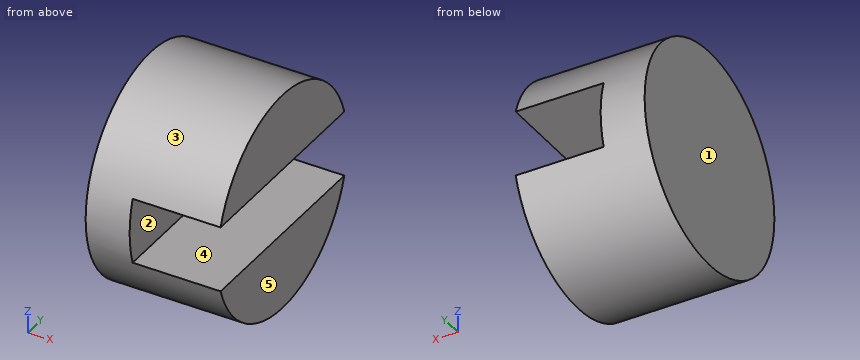
```python
from build123d import *

# Parameters (mm, degrees)
SKETCH2_R           = 5
BOSS_EXTRUDE1_DEPTH = 6
CUT_EXTRUDE1_START  = -4
CUT_EXTRUDE1_DEPTH  = 4


with BuildPart() as part:
    # Sketch2 → Boss-Extrude1 (new body)
    with BuildSketch(Plane(origin=(0, 0, 0), x_dir=(0, 0, -1), z_dir=(1, 0, 0))):
        Circle(SKETCH2_R)
    extrude(amount=BOSS_EXTRUDE1_DEPTH)

    # Sketch3 → Cut-Extrude1 (cut)
    with BuildSketch(Plane(origin=(6, 0, 0), x_dir=(0, 0, -1), z_dir=(1, 0, 0)).offset(CUT_EXTRUDE1_START)):
        with BuildLine():
            Line((-1.5, 4.769696007), (-1.5, -4.769696007))
            ThreePointArc((-1.5, -4.769696007), (0, -5), (1.5, -4.769696007))
            Line((1.5, -4.769696007), (1.5, 4.769696007))
            ThreePointArc((1.5, 4.769696007), (0, 5), (-1.5, 4.769696007))
        make_face()
    extrude(amount=CUT_EXTRUDE1_DEPTH, mode=Mode.SUBTRACT)


solid = part.part
```
Verification items for the finished model (mm, model axes). Face numbers are marked on the shaded views. A direction names the side the tool comes from. Coordinates: 2 decimals unless noted, no trailing zeros. Write each loop counter-clockwise with the first axis right and the second up, starting at its lowest first coordinate (ties: lowest second). Pieces come first, ordered by that corner, then holes. Notation, with made-up numbers: (-12, -25) - (-3, -25) arc R27 cw to (-3, 6) - close; hole circle Ø1 at (20.5, -38). An arc over 180 degrees is marked (long way). One line per question, with ' | ' between items. Start each with the question number.
1. Section check C-C (z = 0). Enter the section's corners in (x, y).
2. Section check D-D (y = 3). Enter the section's corners in (x, z), plus the area to 3 significant figures.
3. Material ranges on line 1 along Z through (x, y) = (5.1, 0); line 2 along X through (y, z) = (3.5, -1); line 3 along Y through (x, z) = (1.25, -1.5), recorded low to high.
4. Gauge pin test, flat ends, axial feed: P1, Ø1.5, axis at x = 4.5, y = -3.5, coming from the -Z side; P2, Ø3, axis at x = 4.5, y = -2, coming from the +Z side; P3, Ø1, axis at x = 3, z = 3.5, coming from the +Y side. Record the tip position at first contact, or that the pin passes through.
5. Draft check along Z on the marked faces 1, 2 and 3. Enter one of: released by +Z, released by -Z, zero draft, split by the parting line, or undercut.
6. Section check B-B (x = 3.35). Enter the section's corners in (y, z), plus the area to 3 significant figures.
7. Access from +Z, -Z, +X, -X, +Y, -Y to the whole of each face (thin tool, end or side, straight path). Record for the marked faces 4 and 5.
8. Section check A-A (y = -4). Enter the section's corners in (x, z), plus the area to 3 significant figures.
Computed values:
1) outline: (0, -5) - (2, -5) - (2, 5) - (0, 5) - close
2) outline: (0, -4) - (6, -4) - (6, -1.5) - (2, -1.5) - (2, 1.5) - (6, 1.5) - (6, 4) - (0, 4) - close | area: 36.0 mm²
3) line 1: -5 to -1.5, 1.5 to 5 | line 2: 0 to 2 | line 3: -4.77 to 4.77
4) P1: z = -4.18 | P2: z = 4.97 | P3: y = 4
5) face 1: zero draft | face 2: undercut | face 3: split by the parting line
6) outline: (-4.77, -1.5) arc R5 ccw to (4.77, -1.5) - close; (-4.77, 1.5) - (4.77, 1.5) arc R5 ccw to start | area: 49.0 mm²
7) face 4: +X, +Y, -Y | face 5: +Z, -Z, +X, +Y, -Y
8) outline: (0, -3) - (6, -3) - (6, -1.5) - (2, -1.5) - (2, 1.5) - (6, 1.5) - (6, 3) - (0, 3) - close | area: 24.0 mm²
